from build123d import *

# Parameters (mm, degrees)
SKETCH2_R           = 50.8
BOSS_EXTRUDE1_DEPTH = 101.6
SKETCH3_R           = 47.625
CUT_EXTRUDE1_DEPTH  = 101.6
SKETCH9_W           = 2921
SKETCH9_H           = 1905
CUT_EXTRUDE4_DEPTH  = 1828.8
SKETCH10_W          = 2914.398267979
SKETCH10_H          = 1269.930665489
CUT_EXTRUDE7_DEPTH  = 508
SKETCH11_W          = 281.911463331
SKETCH11_H          = 233.276474331
CUT_EXTRUDE8_DEPTH  = 153.4


with BuildPart() as part:
    # Sketch2 → Boss-Extrude1 (new body, symmetric)
    with BuildSketch(Plane(origin=(0, 0, 0), x_dir=(0, 0, -1), z_dir=(1, 0, 0))):
        Circle(SKETCH2_R)
    extrude(amount=BOSS_EXTRUDE1_DEPTH, both=True)

    # Sketch3 → Cut-Extrude1 (cut, symmetric)
    with BuildSketch(Plane(origin=(0, 0, 0), x_dir=(0, 0, -1), z_dir=(1, 0, 0))):
        Circle(SKETCH3_R)
    extrude(amount=CUT_EXTRUDE1_DEPTH, both=True, mode=Mode.SUBTRACT)

    # Sketch4 → Revolve-Thin1 (revolve)
    with BuildSketch(Plane.XY):
        with BuildLine():
            ThreePointArc((-101.6, 50.8), (-137.521024484, 35.921024484), (-152.4, 0))
            Line((-152.4, 0), (-149.225, 0))
            ThreePointArc((-149.225, 0), (-135.275960454, 33.675960454), (-101.6, 47.625))
            Line((-101.6, 47.625), (-101.6, 50.8))
        make_face()
    revolve(axis=Axis((-152.4, 0, 0), (1, 0, 0)))

    # Sketch5 → Revolve-Thin2 (revolve)
    with BuildSketch(Plane.XY):
        with BuildLine():
            ThreePointArc((101.6, 50.8), (137.521024484, 35.921024484), (152.4, 0))
            Line((152.4, 0), (149.225, 0))
            ThreePointArc((149.225, 0), (135.275960454, 33.675960454), (101.6, 47.625))
            Line((101.6, 47.625), (101.6, 50.8))
        make_face()
    revolve(axis=Axis((152.4, 0, 0), (-1, 0, 0)))

    # Sketch9 → Cut-Extrude4 (cut)
    with BuildSketch(Plane.XY):
        with Locations((975.277240458, -31.313733989)):
            Rectangle(SKETCH9_W, SKETCH9_H)
    extrude(amount=-CUT_EXTRUDE4_DEPTH, mode=Mode.SUBTRACT)

    # Sketch10 → Cut-Extrude7 (cut)
    with BuildSketch(Plane(origin=(0, 0, 0), x_dir=(1, 0, 0), z_dir=(0, 1, 0))):
        with Locations((902.969453076, -134.938526822)):
            Rectangle(SKETCH10_W, SKETCH10_H)
    extrude(amount=-CUT_EXTRUDE7_DEPTH, mode=Mode.SUBTRACT)

    # Sketch11 → Cut-Extrude8 (cut, through all)
    with BuildSketch(Plane(origin=(0, 0, 0), x_dir=(0, 0, -1), z_dir=(1, 0, 0))):
        with Locations((-43.809030365, 33.571989562)):
            Rectangle(SKETCH11_W, SKETCH11_H)
    extrude(amount=-CUT_EXTRUDE8_DEPTH, mode=Mode.SUBTRACT)


solid = part.part
The listing builds one solid part. Answer for the finished solid, in the listing's coordinates (mm). A direction names the side the tool comes from. Round coordinates to 2 decimals unless told otherwise and drop trailing zeros. Order: outer loops, then holes, each group sorted by start corner. A loop starts at its lowest first (then second) coordinate and runs counter-clockwise, first axis right, second up. Notation, with made-up numbers: (75, 59.25) -> (101, 59.25) arc R32 ccw to (101, 88.25) -> close; hole circle Ø7 at (-29.5, -37). An arc over 180 degrees is marked (long way). One line per item, written item: value.
Item 1: Given P1, Ø2, axis at x = 86.5, y = 36, coming from the +Z side; P2, Ø8, axis at x = 22, z = 35, coming from the +Y side; P3, Ø2, axis at x = 51, y = 35.5, coming from the -Z side, each flat-ended and moving along its own axis, determine where each tip first touches the part or whether it passes through.
Taken from the geometry:
P1: stops at z = 36.82
P2: stops at y = 40.24
P3: stops at z = 30.59
Item 2: For faces 1 (the cylindrical face through (51.511, 36.314, 35.524)), 2 (the cylindrical face through (51.511, 34.044, 33.304)), determine the directions among +Z, -Z, +X, -X, +Y, -Y from which every point of the face is accessible in a straight line to the end or side of a thin tool.
Taken from the geometry:
face 1: +Z, +X, -X, +Y
face 2: -Z, -X, -Y
Item 3: Straight lines are drawn through the part: L1, parallel to Z at x = 91.5, y = 28; L2, parallel to X at y = 18, z = 16; L3, parallel to Y at x = 62.5, z = 20. For each, find the intervals that lie inside material, in ascending order.
Taken from the geometry:
L1: z = 38.52 to 42.39
L2: x = 142.69 to 146.33
L3: y = 43.22 to 46.7
Item 4: Find section C-C, the plane x = 94.5. Give the vertices of the cut face in (y, z) (3 decimals), then the cut area to 3 significant figures.
Taken from the geometry:
outline: (0, 47.625) arc R47.625 cw to (47.625, 0) -> (50.8, 0) arc R50.8 ccw to (0, 50.8) -> close
area: 245 mm2
Item 5: Find section B-B, the plane z = 45. Give the vertices of the cut face in (x, y), then the cut area to 3 significant figures.
Taken from the geometry:
outline: (0, 15.59) -> (101.6, 15.59) arc R15.59 cw to (117.19, 0) -> (125.17, 0) arc R23.57 ccw to (101.6, 23.57) -> (0, 23.57) -> close
area: 1,060 mm2
Item 6: Find section A-A, the plane y = 6.5. Give the vertices of the cut face in (x, z).
Taken from the geometry:
outline: (0, 47.18) -> (101.6, 47.18) arc R47.18 cw to (148.78, 0) -> (151.98, 0) arc R50.38 ccw to (101.6, 50.38) -> (0, 50.38) -> close
